Geometry check sheet. Reference: the model listing, model coordinates, mm. Face numbers are marked on the shaded views. A direction names the side the tool comes from. Give positions to 0.01 mm unless a question says otherwise; leave off trailing zeros. Loops run counter-clockwise (first coordinate to the right, second up) from the corner with the lowest first, then second, coordinate; pieces in that order, holes last. Notation, with made-up numbers: (73.25, 60) -> (116.25, 60) arc R23 cw to (116.25, 98) -> close; hole circle Ø9 at (-10, -4). An arc over 180 degrees is marked (long way). One line per item, written item: value. Start each with the question number.
(1) Scan lines: line 1 along X through (y, z) = (-12.2, 0); line 2 along Y through (x, z) = (29.5, 3.75); line 3 along Z through (x, y) = (7.5, 12.9). Record each from-to range of solid material in increasing order. Write a range as from..to.
(2) Sectioned sample at D-D, the plane y = 6.5. Record the cut outline in (x, z).
(3) Sectioned sample at C-C, the plane z = 0. Record the cut outline in (x, y).
(4) Sectioned sample at B-B, the plane x = 7.5. Record the cut outline in (y, z).
(5) Gauge pin test, flat ends, axial feed: pin 1 Ø5 at (x, z) = (7.5, 0) entering from -Y; pin 2 Ø6 at (x, y) = (27.5, 5.5) entering from -Z; pin 3 Ø16 at (x, y) = (20.5, 3.5) entering from -Z. Record the tip position at first contact, or that the pin passes through.
(6) Tool access check on the marked faces 1, 2 and 3. Record the directions out of +Z, -Z, +X, -X, +Y, -Y that give a thin tool (end or side, any length) a straight path to the whole face; none if there is none.
(7) Sectioned sample at A-A, the plane z = 7.75. Record the cut outline in (x, y), then the cut area to 3 significant figures.
(8) Draft check along X on the marked faces 4, 5 and 6. Enter one of: pulls with the +X half, pulls with the -X half, needs draft (parallel to the pull), parting line crosses it, or undercut.
from build123d import *

# Parameters (mm, degrees)
BOSS_EXTRUDE1_DEPTH = 40
SKETCH5_R           = 2.7
CUT_EXTRUDE1_DEPTH  = 31.1


with BuildPart() as part:
    # Sketch1 → Boss-Extrude1 (new body)
    with BuildSketch(Plane(origin=(0, 0, 0), x_dir=(0, 0, -1), z_dir=(1, 0, 0))):
        Polygon((10.05, -10.05), (10.05, -15.05), (-15.05, -15.05), (-15.05, 15.05), (10.05, 15.05), (10.05, 10.05), (-10.05, 10.05), (-10.05, -10.05), align=None)
    extrude(amount=BOSS_EXTRUDE1_DEPTH)

    # Sketch5 → Cut-Extrude1 (cut, through all)
    with BuildSketch(Plane(origin=(0, 15.05, 0), x_dir=(1, 0, 0), z_dir=(0, 1, 0))):
        with Locations((7.5, 0)):
            Circle(SKETCH5_R)
        with Locations((26.5, 0)):
            Circle(SKETCH5_R)
        Polygon((34, -15.05), (36.5, -12.05), (39, -15.05), align=None)
        Polygon((36.5, 7.05), (39, 10.05), (34, 10.05), align=None)
    extrude(amount=-CUT_EXTRUDE1_DEPTH, mode=Mode.SUBTRACT)


solid = part.part
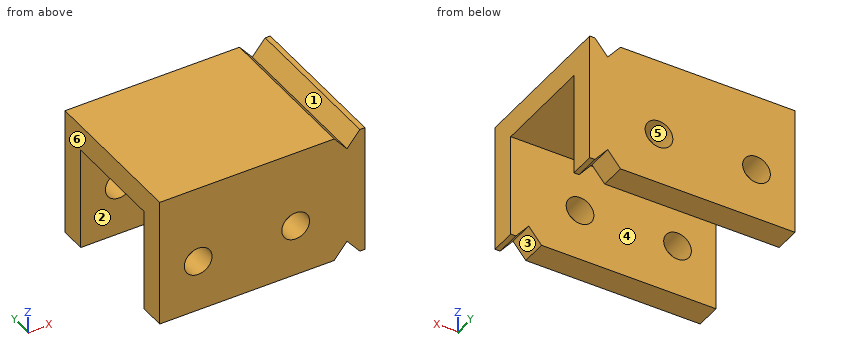
Calculated:
1. line 1: x = 0..4.8, 10.2..23.8, 29.2..40
1. line 2: y = -15.05..-10.05, 10.05..15.05
1. line 3: z = -10.05..-2.7, 2.7..15.05
2. outline: (0, 10.05) -> (40, 10.05) -> (40, 15.05) -> (39, 15.05) -> (36.5, 12.05) -> (34, 15.05) -> (0, 15.05) -> close
3. outline: (0, -15.05) -> (4.8, -15.05) -> (4.8, -10.05) -> (0, -10.05) -> close; (0, 10.05) -> (4.8, 10.05) -> (4.8, 15.05) -> (0, 15.05) -> close; (10.2, -15.05) -> (23.8, -15.05) -> (23.8, -10.05) -> (10.2, -10.05) -> close; (10.2, 10.05) -> (23.8, 10.05) -> (23.8, 15.05) -> (10.2, 15.05) -> close; (29.2, -15.05) -> (40, -15.05) -> (40, -10.05) -> (29.2, -10.05) -> close; (29.2, 10.05) -> (40, 10.05) -> (40, 15.05) -> (29.2, 15.05) -> close
4. outline: (-15.05, -10.05) -> (-10.05, -10.05) -> (-10.05, -2.7) -> (-15.05, -2.7) -> close; (-15.05, 2.7) -> (-10.05, 2.7) -> (-10.05, 10.05) -> (10.05, 10.05) -> (10.05, 2.7) -> (15.05, 2.7) -> (15.05, 15.05) -> (-15.05, 15.05) -> close; (10.05, -10.05) -> (15.05, -10.05) -> (15.05, -2.7) -> (10.05, -2.7) -> close
5. pin 1: passes through
5. pin 2: stops at z = 10.05
5. pin 3: stops at z = -10.05
6. face 1: +Z, +Y, -Y
6. face 2: -Z, +X, -X
6. face 3: -Z, +Y, -Y
7. outline: (0, -15.05) -> (40, -15.05) -> (40, -10.05) -> (0, -10.05) -> close; (0, 10.05) -> (40, 10.05) -> (40, 15.05) -> (0, 15.05) -> close
7. area: 400 mm2
8. face 4: needs draft
8. face 5: undercut
8. face 6: pulls with the -X half
